Could you check a few things on this drawing? It's one solid part, dimensions in mm from its lowest x, y, z. A direction names the side the tool comes from. Coordinates: 2 decimals unless noted, no trailing zeros. Write each loop counter-clockwise with the first axis right and the second up, starting at its lowest first coordinate (ties: lowest second). Pieces come first, ordered by that corner, then holes. Notation, with made-up numbers: (-19, 46) - (-11, 46) arc R15 cw to (-11, 60) - close; hole circle Ø5 at (-15.5, -31). An arc over 180 degrees is marked (long way). Write item = value, one per line. Start each with the question number.
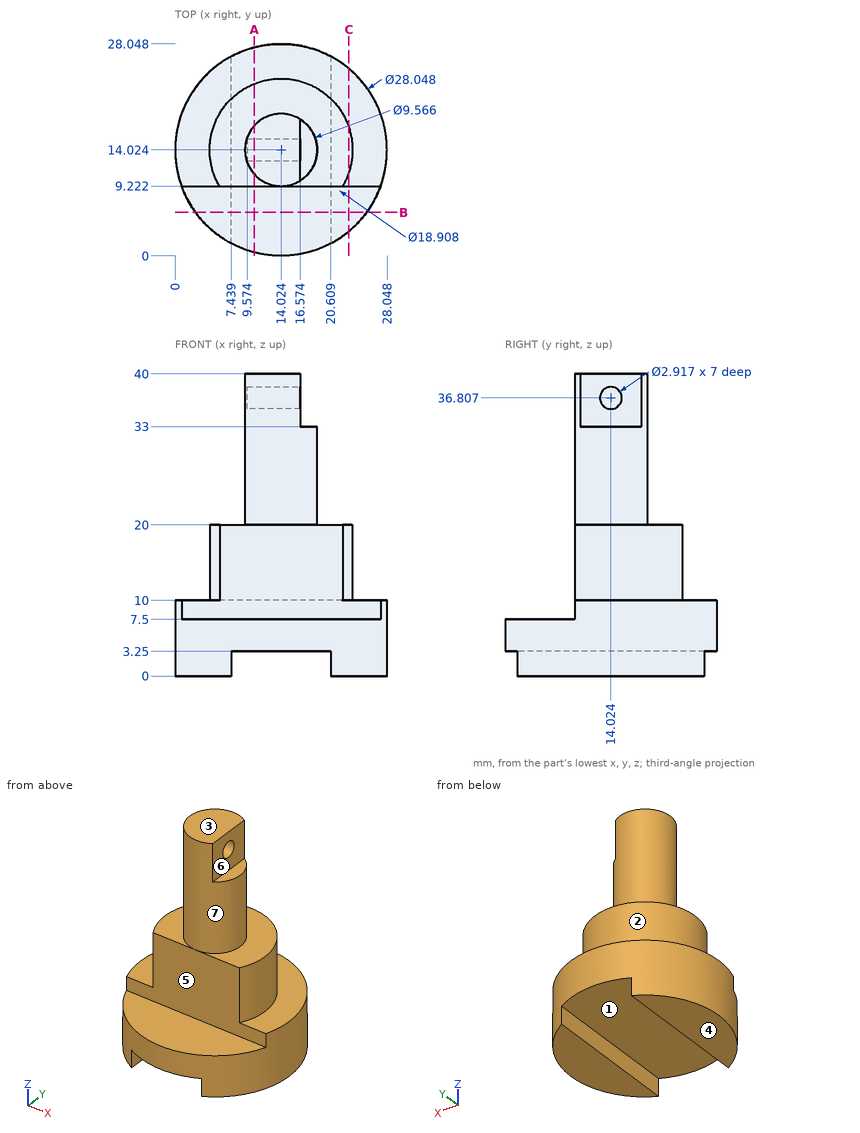
1) Suppose I cut it at B-B on y = 5.75. Please give me the cut outline in (x, z).
2) Suppose I cut it at C-C on x = 23. Please give me the cut outline in (y, z).
3) Suppose I cut it at A-A on x = 10.5. Please give me the cut outline in (y, z), plus the area to 3 significant figures.
4) Which directions (+Z, -Z, +X, -X, +Y, -Y) give clear straight access to the entire face, cutting with the end or side of a thin tool? Please do the marked faces 4, 5, 6 and 7.
5) Thinking about a two-plate mould opening in X: for the marked faces 1, 2 and 3, which applies, +X half, -X half, draft (parallel to the pull), parting line (faces both ways), or undercut?
6) If I drill on probe 1 along Z at (x, y) = (12.75, 18); probe 2 along Z at (x, y) = (5.5, 14.5); probe 3 along Y at (x, z) = (10.5, 36), over which ranges is the centre line in solid material (lowest first)? Write a range as [from, to].
7) For P1, Ø8, axis at y = 20.5, z = 6.5, coming from the -X side; P2, Ø1.5, axis at x = 25, z = 13.5, coming from the -Y side; P3, Ø1, axis at y = 15, z = 1, coming from the +X side; P4, Ø2.5, axis at x = 18, y = 15.5, coming from the +Z side, each with a flat end and sliding along its axis, tell me the tip position at first contact or that it passes through.
Reply:
q1.outline = (2.7, 0) - (7.44, 0) - (7.44, 3.25) - (20.61, 3.25) - (20.61, 0) - (25.35, 0) - (25.35, 7.5) - (2.7, 7.5) - close
q2.outline = (3.25, 0) - (24.8, 0) - (24.8, 10) - (16.99, 10) - (16.99, 20) - (11.06, 20) - (11.06, 10) - (9.22, 10) - (9.22, 7.5) - (3.25, 7.5) - close
q3.outline = (0.45, 3.25) - (27.6, 3.25) - (27.6, 10) - (22.8, 10) - (22.8, 20) - (17.26, 20) - (17.26, 40) - (10.79, 40) - (10.79, 20) - (9.22, 20) - (9.22, 7.5) - (0.45, 7.5) - close; hole circle Ø2.92 at (14.02, 36.81)
q3.area = 420 mm^2
q4.face_4 = -Z, +X, -X, +Y, -Y
q4.face_5 = +Z, +X, -X, -Y
q4.face_6 = +Z, +X, +Y, -Y
q4.face_7 = +Z
q5.face_1 = undercut
q5.face_2 = parting line
q5.face_3 = draft
q6.probe_1 = [3.25, 40]
q6.probe_2 = [0, 20]
q6.probe_3 = [10.79, 12.81], [15.24, 17.26]
q7.P1 = 0.22
q7.P2 = through
q7.P3 = 28.04
q7.P4 = 33
